Build history of the part. All positions in model axes, mm. A direction names the side the tool comes from. Give positions to 0.01 mm unless a question says otherwise; leave off trailing zeros. Order: outer loops, then holes, each group sorted by start corner. A loop starts at its lowest first (then second) coordinate and runs counter-clockwise, first axis right, second up. Notation, with made-up numbers: (4, 71) -> (38, 71) arc R32 cw to (38, 107) -> close; hole circle Ø3 at (-34, 86). An arc over 180 degrees is marked (long way). One line per question, with ' | ' between items. Start each with the question number.
(1) Pull direction Z, two halves, no side cores. Call faces 3 (the face through (45.105, 1.479, -34.318)), 4 (the face through (1, 1, 36.83)), 5 (the face through (44, 1, 0)): +Z half, -Z half, draft (parallel to the pull), parting line (faces both ways), or undercut.
(2) Cut at C-C (y = 1). Give the cut face in (x, z).
(3) Cut at A-A (z = 19). Give the cut face in (x, y).
(4) Cut at B-B (x = 8). Give the cut face in (y, z), then the cut area to 3 significant figures.
(5) Which spindle directions (+Z, -Z, +X, -X, +Y, -Y) get a long thin tool onto all of the face, cutting with end or side? Do faces 1 (the face through (-45, 1.5, -34.2)), 2 (the face through (-37.18, 1.48, -26.56)). Say none if no direction does.
(6) Drill centre lines: L1, parallel to Z at x = -11, y = 1.2; L2, parallel to X at y = 1.9, z = -14; L3, parallel to X at y = 1.95, z = 28.5. Where is each one in solid material? Low to high. Write a range as from..to.
(7) Pin check, flat tip, straight feed: pin 1 Ø2 at (x, z) = (-39.89, -29.67) entering from -Y. Stop position of the tip, or through.
from build123d import *

# Parameters (mm, degrees)
IZIM1_R                     = 1.8
Y_KSEKLIK_EKSTR_ZYON1_DEPTH = 3


with BuildPart() as part:
    # Çizim1 → Yükseklik-Ekstrüzyon1 (new body)
    with BuildSketch(Plane(origin=(0, 0, 0), x_dir=(1, 0, 0), z_dir=(0, 1, 0))):
        with BuildLine():
            Line((-37.887405356, 37.169798919), (38.112594644, 37.169798919))
            ThreePointArc((38.112594644, 37.169798919), (45.183662456, 34.240866731), (48.112594644, 27.169798919))
            Line((48.112594644, 27.169798919), (48.112594644, -26.830201081))
            ThreePointArc((48.112594644, -26.830201081), (45.183662456, -33.901268893), (38.112594644, -36.830201081))
            Line((38.112594644, -36.830201081), (-37.887405356, -36.830201081))
            ThreePointArc((-37.887405356, -36.830201081), (-44.958473168, -33.901268893), (-47.887405356, -26.830201081))
            Line((-47.887405356, -26.830201081), (-47.887405356, 27.169798919))
            ThreePointArc((-47.887405356, 27.169798919), (-44.958473168, 34.240866731), (-37.887405356, 37.169798919))
        make_face()
        with Locations(Location((-39.887405356, 29.669798919, 0), (0, 0, 270))):
            Circle(IZIM1_R, mode=Mode.SUBTRACT)
        with Locations(Location((40.112594644, 29.669798919, 0), (0, 0, 270))):
            Circle(IZIM1_R, mode=Mode.SUBTRACT)
        with Locations(Location((-39.887405356, -29.330201081, 0), (0, 0, 270))):
            Circle(IZIM1_R, mode=Mode.SUBTRACT)
        with Locations(Location((40.112594644, -29.330201081, 0), (0, 0, 270))):
            Circle(IZIM1_R, mode=Mode.SUBTRACT)
        with BuildLine():
            Line((-44, 20.5), (-44, -20.5))
            ThreePointArc((-44, -20.5), (-42.535533906, -24.035533906), (-39, -25.5))
            ThreePointArc((-39, -25.5), (-36.935561042, -26.597935324), (-35.837625718, -28.662374282))
            ThreePointArc((-35.837625718, -28.662374282), (-34.373159624, -32.197908188), (-30.837625718, -33.662374282))
            Line((-30.837625718, -33.662374282), (31.162374282, -33.662374282))
            ThreePointArc((31.162374282, -33.662374282), (34.697908188, -32.197908188), (36.162374282, -28.662374282))
            ThreePointArc((36.162374282, -28.662374282), (37.138980167, -26.684391009), (39, -25.5))
            ThreePointArc((39, -25.5), (42.535533906, -24.035533906), (44, -20.5))
            Line((44, -20.5), (44, 20.5))
            ThreePointArc((44, 20.5), (42.535533906, 24.035533906), (39, 25.5))
            ThreePointArc((39, 25.5), (37.03578822, 26.490091983), (35.866325447, 28.353091412))
            ThreePointArc((35.866325447, 28.353091412), (34.401859353, 31.888625318), (30.866325447, 33.353091412))
            Line((30.866325447, 33.353091412), (-31.133674553, 33.353091412))
            ThreePointArc((-31.133674553, 33.353091412), (-34.677536648, 31.880277464), (-36.133618935, 28.329507991))
            ThreePointArc((-36.133618935, 28.329507991), (-37.197839579, 26.540975831), (-39, 25.5))
            ThreePointArc((-39, 25.5), (-42.535533906, 24.035533906), (-44, 20.5))
        make_face(mode=Mode.SUBTRACT)
    extrude(amount=Y_KSEKLIK_EKSTR_ZYON1_DEPTH)


solid = part.part
Result set:
1) face 3: -Z half | face 4: +Z half | face 5: undercut
2) outline: (-47.89, -27.17) arc R10 ccw to (-37.89, -37.17) -> (38.11, -37.17) arc R10 ccw to (48.11, -27.17) -> (48.11, 26.83) arc R10 ccw to (38.11, 36.83) -> (-37.89, 36.83) arc R10 ccw to (-47.89, 26.83) -> close; hole (-44, -20.5) arc R5 ccw to (-39, -25.5) arc R4.12 cw to (-36.13, -28.33) arc R5 ccw to (-31.13, -33.35) -> (30.87, -33.35) arc R5 ccw to (35.87, -28.35) arc R4.1 cw to (39, -25.5) arc R5 ccw to (44, -20.5) -> (44, 20.5) arc R5 ccw to (39, 25.5) arc R4.1 cw to (36.16, 28.66) arc R5 ccw to (31.16, 33.66) -> (-30.84, 33.66) arc R5 ccw to (-35.84, 28.66) arc R4 cw to (-39, 25.5) arc R5 ccw to (-44, 20.5) -> close; hole circle Ø3.6 at (-39.89, -29.67); hole circle Ø3.6 at (-39.89, 29.33); hole circle Ø3.6 at (40.11, -29.67); hole circle Ø3.6 at (40.11, 29.33)
3) outline: (-47.89, 0) -> (-44, 0) -> (-44, 3) -> (-47.89, 3) -> close; (44, 0) -> (48.11, 0) -> (48.11, 3) -> (44, 3) -> close
4) outline: (0, -37.17) -> (3, -37.17) -> (3, -33.35) -> (0, -33.35) -> close; (0, 33.66) -> (3, 33.66) -> (3, 36.83) -> (0, 36.83) -> close | area: 21.0 mm2
5) face 1: -Z, -X, +Y, -Y | face 2: +Y, -Y
6) L1: z = -37.17..-33.35, 33.66..36.83 | L2: x = -47.89..-44, 44..48.11 | L3: x = -47.75..-41.48, -38.29..-35.87, 36.2..38.52, 41.71..47.97
7) pin 1: passes through
